```python
from build123d import *

# Parameters (mm, degrees)
F0_W     = 67.31
F0_H     = 138.43
F1_DEPTH = 7.366
F2_R     = 5.985409
F2_R_2   = 5.035969
F2_R_3   = 4.859729
F2_R_4   = 4.852246
F2_R_5   = 6.223489
F2_R_6   = 7.822156
F2_R_7   = 7.817507
F2_R_8   = 2.695695
F3_DEPTH = 25.4
F5_DEPTH = 25.4


with BuildPart() as f1:
    # F0 (on Front) → F1 (new body)
    with BuildSketch(Plane.XZ):
        with Locations((12.122316, 20.691026)):
            Rectangle(F0_W, F0_H)
    extrude(amount=F1_DEPTH)

    # F2 (on face) → F3 (cut)
    with BuildSketch(Plane.XZ.offset(7.366)):
        with Locations((26.417792, 64.943209)):
            Circle(F2_R)
        with Locations((-11.861048, 75.99555)):
            Circle(F2_R_2)
        with Locations((-5.930525, 36.908004)):
            Circle(F2_R_3)
        with Locations((8.087078, 16.690306)):
            Circle(F2_R_4)
        with Locations((27.496068, 12.916337)):
            Circle(F2_R_5)
        with Locations((-7.81751, -5.953513)):
            Circle(F2_R_6)
        with Locations((16.443726, -12.423175)):
            Circle(F2_R_7)
        with Locations((25.878653, 44.186372)):
            Circle(F2_R_8)
    extrude(amount=-F3_DEPTH, mode=Mode.SUBTRACT)

    # F4 (on face) → F5 (cut)
    with BuildSketch(Plane.XZ.offset(7.366)):
        Polygon((17.936366, 32.632034), (5.725363, 45.173392), (17.936366, 25.152631), (22.55336, 27.968614), (39.092198, 17.363565), (22.145992, 32.632034), align=None)
    extrude(amount=-F5_DEPTH, mode=Mode.SUBTRACT)


solid = f1.part
```
The model under review builds one solid part; all positions refer to its coordinate system, in mm. A direction names the side the tool comes from. Round coordinates to 2 decimals unless told otherwise and drop trailing zeros. Loops run counter-clockwise (first coordinate to the right, second up) from the corner with the lowest first, then second, coordinate; pieces in that order, holes last.
Item 1: Take a section at A-A (z = 73). Write out the cut boundary in (x, y), then the cut area to 3 significant figures.
Determined:
outline: (-21.53, -7.37) - (-15.91, -7.37) - (-15.91, 0) - (-21.53, 0) - close; (-7.81, -7.37) - (45.78, -7.37) - (45.78, 0) - (-7.81, 0) - close
area: 436 mm2
Item 2: Mouldability with a two-part tool opening along Z and no side actions: class faces 1 (the face through (7.035, -3.735, 11.953)), 2 (the face through (-21.533, -4, 20)), 3 (the face through (12, -4, 89.906)) as released by +Z, released by -Z, zero draft, split by the parting line, or undercut.
Determined:
face 1: undercut
face 2: zero draft
face 3: released by +Z
Item 3: For line 1 (Z direction, x = -10, y = -6.25); line 2 (Z direction, x = 25, y = -4.25); line 3 (Z direction, x = -2.5, y = -5.25), list the stretches that pass through material, from the lowest coordinate up.
Determined:
line 1: z = -48.52 to -13.47, 1.56 to 34.25, 39.56 to 71.32, 80.68 to 89.91
line 2: z = -48.52 to 7.22, 18.62 to 26.4, 30.06 to 41.64, 46.73 to 59.13, 70.76 to 89.91
line 3: z = -48.52 to -11.69, -0.22 to 33.47, 40.35 to 89.91
Item 4: Take a section at C-C (y = -5.25). Give the number of separate pieces and of enclosed holes in the cut face, then the cut area to 3 significant figures.
Determined:
separate pieces: 1
enclosed holes: 9
area: 8,340 mm2
Item 5: Take a section at B-B (x = -4.5). Write out the cut boundary in (y, z).
Determined:
outline: (-7.37, -48.52) - (0, -48.52) - (0, -13.04) - (-7.37, -13.04) - close; (-7.37, 1.13) - (0, 1.13) - (0, 32.26) - (-7.37, 32.26) - close; (-7.37, 41.55) - (0, 41.55) - (0, 89.91) - (-7.37, 89.91) - close
Item 6: For faces 4 (the face through (12, -4, -48.524)), 5 (the face through (20.21, -3.73, 26.54)), list the 3-axis set-ups (+Z, -Z, +X, -X, +Y, -Y) from which the entire face can be reached by the end or side of a thin tool; tool diameter is ignored.
Determined:
face 4: -Z, +X, -X, +Y, -Y
face 5: +Y, -Y
